The model under review builds one solid part; all positions refer to its coordinate system, in mm. Face numbers are marked on the shaded views. Coordinates: 2 decimals unless noted, no trailing zeros. Write each loop counter-clockwise with the first axis right and the second up, starting at its lowest first coordinate (ties: lowest second). Pieces come first, ordered by that corner, then holes. Notation, with made-up numbers: M 89.5,53 L 106.5,53 A23 cw 106.5,83 Z; hole C -35,45 d4. An arc over 180 degrees is marked long. Answer as CSV lines item,"result". Start each with the question number.
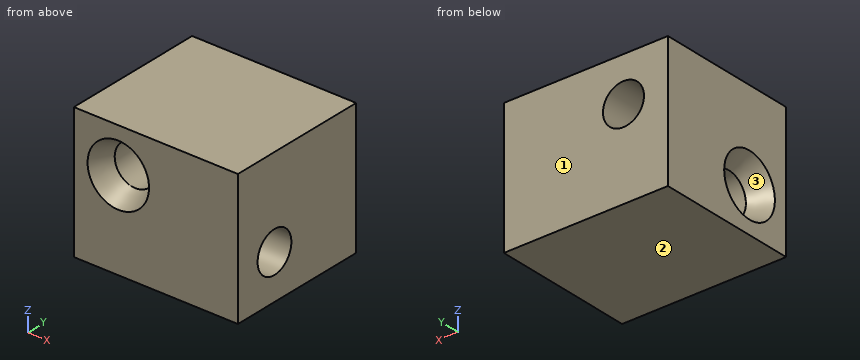
from build123d import *

# Parameters (mm, degrees)
SKETCH_W        = 16
SKETCH_H        = 14
PAD_DEPTH       = 13
SKETCH001_R     = 2
POCKET_DEPTH    = 16.001
SKETCH002_R     = 2
POCKET001_DEPTH = 14.001
CHAMFER_1_SIZE2 = 2
CHAMFER_1_SIZE  = 1
CHAMFER_2_SIZE2 = 2
CHAMFER_2_SIZE  = 1


with BuildPart() as part:
    # Sketch → Pad (new body)
    with BuildSketch(Plane.XY):
        with Locations((8, 7)):
            Rectangle(SKETCH_W, SKETCH_H)
    extrude(amount=PAD_DEPTH)

    # Sketch001 (on Face2 of Pad) → Pocket (cut, through all)
    with BuildSketch(Plane.YZ.offset(16)):
        with Locations((4.333333, 4.333333)):
            Circle(SKETCH001_R)
    extrude(amount=-POCKET_DEPTH, mode=Mode.SUBTRACT)

    # Sketch002 (on Face6 of Pocket) → Pocket001 (cut, through all)
    with BuildSketch(Plane(origin=(0, 14, 0), x_dir=(-1, 0, 0), z_dir=(0, 1, 0))):
        with Locations((-4.333333, 8.666667)):
            Circle(SKETCH002_R)
    extrude(amount=-POCKET001_DEPTH, mode=Mode.SUBTRACT)

    # Chamfer 1
    chamfer_1_edges = [part.edges().sort_by_distance(p)[0] for p in [
        (6.333333, 0, 8.666667),
    ]]
    chamfer_1_side = part.faces().sort_by_distance((8.235766, 0, 6.360683))[0]
    chamfer(chamfer_1_edges, length=CHAMFER_1_SIZE, length2=CHAMFER_1_SIZE2, reference=chamfer_1_side)

    # Chamfer 2
    chamfer_2_edges = [part.edges().sort_by_distance(p)[0] for p in [
        (0, 2.333333, 4.333333),
    ]]
    chamfer_2_side = part.faces().sort_by_distance((0, 7.197778, 6.660695))[0]
    chamfer(chamfer_2_edges, length=CHAMFER_2_SIZE, length2=CHAMFER_2_SIZE2, reference=chamfer_2_side)


solid = part.part
1) To check wall thickness, follow line 1 (Z direction, x = 2.5, y = 6); line 2 (Z direction, x = 3.25, y = 5.5); line 3 (Y direction, x = 6.5, z = 6). State the ranges of each line that lie inside material, in increasing order. Write a range as [from, to].
2) Take a section at D-D on y = 11.75. Give the boundary of the cut face in (x, z), and give its area (3 significant figures).
3) Clearance check with a flat-ended pin moving along its axis: pin 1 Ø2.5 at (y, z) = (4.33, 4.33) entering from -X. State where the tip first meets the part, or that it passes through.
4) Take a section at C-C on x = 14.5. Give the boundary of the cut face in (y, z).
5) Take a section at A-A on x = 4.5. Give the number of separate pieces and of enclosed holes in the cut face, and give its area (3 significant figures).
6) Mouldability with a two-part tool opening along Z and no side actions: class the marked faces 1, 2 and 3 as +Z half, -Z half, draft (parallel to the pull), parting line (faces both ways), or undercut.
Results:
1,line 1,"z = [0, 3.23], [5.44, 7.87], [9.47, 13]"
1,line 2,"z = [0, 2.71], [5.96, 6.99], [10.35, 13]"
1,line 3,"y = [0, 3.23], [5.44, 14]"
2,outline,"M 0,0 L 16,0 L 16,13 L 0,13 Z; hole C 4.33,8.67 d4"
2,area,"195 mm²"
3,pin 1,"passes through"
4,outline,"M 0,0 L 14,0 L 14,13 L 0,13 Z; hole C 4.33,4.33 d4"
5,separate pieces,"2"
5,enclosed holes,"1"
5,area,"112 mm²"
6,face 1,"draft"
6,face 2,"-Z half"
6,face 3,"undercut"
